Work out the finished part from the listing and answer in its coordinate system (mm). A direction names the side the tool comes from. Give positions to 0.01 mm unless a question says otherwise; leave off trailing zeros. Order: outer loops, then holes, each group sorted by start corner. A loop starts at its lowest first (then second) coordinate and runs counter-clockwise, first axis right, second up. Notation, with made-up numbers: M 36.5,-36.75 L 58.5,-36.75 A4 ccw 58.5,-29.75 Z; hole C -31.5,-10 d2. An arc over 180 degrees is marked long. One line per item, written item: value.
from build123d import *

# Parameters (mm, degrees)
BOSS_EXTRUDE1_DEPTH = 400


with BuildPart() as part:
    # Sketch1 → Boss-Extrude1 (new body)
    with BuildSketch(Plane(origin=(0, 0, 0), x_dir=(0, 0, -1), z_dir=(1, 0, 0))):
        with BuildLine():
            Line((5, -5), (5, -125.270799085))
            Line((5, -125.270799085), (235, -125.270799085))
            Line((235, -125.270799085), (235, -5))
            Line((235, -5), (235, 4.729200915))
            ThreePointArc((235, 4.729200915), (235.234314575, 5.29488634), (235.8, 5.529200915))
            Line((235.8, 5.529200915), (255.315878667, 5.529200915))
            Line((255.315878667, 5.529200915), (255.315878667, 0.529200915))
            Line((255.315878667, 0.529200915), (240.770883182, -0.000530044))
            ThreePointArc((240.770883182, -0.000530044), (240.224112227, -0.244704337), (240, -0.8))
            Line((240, -0.8), (240, -130.270799085))
            Line((240, -130.270799085), (0, -130.270799085))
            Line((0, -130.270799085), (0, -0.270799085))
            ThreePointArc((0, -0.270799085), (-0.234314575, 0.29488634), (-0.8, 0.529200915))
            Line((-0.8, 0.529200915), (-15.315878667, 0.529200915))
            Line((-15.315878667, 0.529200915), (-15.315878667, 5.529200915))
            Line((-15.315878667, 5.529200915), (4.2, 5.529200915))
            ThreePointArc((4.2, 5.529200915), (4.765685425, 5.29488634), (5, 4.729200915))
            Line((5, 4.729200915), (5, -5))
        make_face()
    extrude(amount=BOSS_EXTRUDE1_DEPTH)


solid = part.part
(1) Section C-C, the plane z = -128.5 is taken. Give the vertices of the cut face in (x, y).
Findings:
outline: M 0,-130.27 L 400,-130.27 L 400,-125.27 L 0,-125.27 Z
(2) Determine the mould class of faces 1 (the flat face through (197.2, 0.27, -248.15)), 2 (the flat face through (197, -66, 0)), 3 (the flat face through (197, -59, -5)), 4 (the flat face through (197, -130.271, -122)) for opening direction Z: pulls with the +Z half, pulls with the -Z half, needs draft (parallel to the pull), parting line crosses it, or undercut.
Findings:
face 1: pulls with the -Z half
face 2: pulls with the +Z half
face 3: undercut
face 4: needs draft
(3) Find the intervals of material crossed by probe 1 along Z at (x, y) = (104.5, -24.5); probe 2 along Y at (x, z) = (118, -22), in increasing order. Write a range as from..to.
Findings:
probe 1: z = -240..-235, -5..0
probe 2: y = -130.27..-125.27
(4) Section B-B, the plane x = 347 is taken. Give the vertices of the cut face in (y, z).
Findings:
outline: M -130.27,-240 L -0.8,-240 A0.8 cw 0,-240.77 L 0.53,-255.32 L 5.53,-255.32 L 5.53,-235.8 A0.8 ccw 4.73,-235 L -125.27,-235 L -125.27,-5 L 4.73,-5 A0.8 ccw 5.53,-4.2 L 5.53,15.32 L 0.53,15.32 L 0.53,0.8 A0.8 cw -0.27,0 L -130.27,0 Z
(5) Given P1, Ø1.5, axis at x = 341, y = -16, coming from the -Z side; P2, Ø3, axis at x = 346, y = -18, coming from the +Z side; P3, Ø7.5, axis at x = 119.5, z = 6, coming from the -Y side, each flat-ended and moving along its own axis, determine where each tip first touches the part or whether it passes through.
Findings:
P1: stops at z = -240
P2: stops at z = 0
P3: stops at y = 0.53
(6) Section A-A, the plane y = -50 is taken. Give the vertices of the cut face in (x, z).
Findings:
outline: M 0,-240 L 400,-240 L 400,-235 L 0,-235 Z; M 0,-5 L 400,-5 L 400,0 L 0,0 Z
(7) Which of the six approach directions +Z, -Z, +X, -X, +Y, -Y give full straight-line access (tool end or side, diameter ignored) to faces 5 (the flat face through (197, 0.529, 8)), 6 (the flat face through (197, -61, -235)), 7 (the flat face through (197, -65, -240))?
Findings:
face 5: +Z, +X, -X, -Y
face 6: +X, -X, +Y
face 7: -Z, +X, -X, -Y
